Input: part model. Units: mm. Frame: model coordinates. A direction names the side the tool comes from. Round coordinates to 2 decimals unless told otherwise and drop trailing zeros. Loops run counter-clockwise (first coordinate to the right, second up) from the corner with the lowest first, then second, coordinate; pieces in that order, holes last. Notation, with made-up numbers: (38.5, 21) -> (61.5, 21) arc R25 ccw to (61.5, 37) -> close; hole circle Ø5 at (-34, -8.5). An arc over 180 degrees is marked (long way). Answer as a JSON object with one key per item and string values. Group by question number.
Item 1: Section query A-A on z = 0. Count the separate pieces of the cut face and the enclosed holes in it, and give its area (3 significant figures).
Item 2: Section query D-D on z = 2. Return loops of the section in (x, y).
Item 3: Section query C-C on x = 0.75. Return loops of the section in (y, z).
Item 4: Pin query (flat end, axial travel): pin 1 (1 mm diameter, centred on x = 3, z = -3, fed in from +Y); pin 2 (1.3 mm diameter, centred on x = -3.5, y = 5, fed in from +Z); pin 3 (2.5 mm diameter, centred on x = -2.5, z = 0, fed in from +Y). Return the tip coordinate at first contact, or that it passes through.
Item 5: Section query B-B on y = 3. Return loops of the section in (x, z), and give its area (3 significant figures).
Item 6: Draft query along Z for faces 4 (the flat face through (-5.004, 5, 0)), 5 (the flat face through (-2, 7.468, 0)), 6 (the cylindrical face through (3.144, -1.252, 0.084)). Return one class per face: released by +Z, released by -Z, zero draft, split by the parting line, or undercut.
Item 7: Material intervals for line 1 (X direction, y = 3.25, z = 0); line 2 (Y direction, x = 4.5, z = 1); line 3 (Y direction, x = -3.5, z = 0), sorted ascending. Write a range as [from, to].
Item 8: Set-up query: faces 1 (the flat face through (2, 6.604, 1)), 2 (the cylindrical face through (4.013, 8.755, -0.198)), 3 (the flat face through (-0.07, 8.45, 3.05)). Return all of +Z, -Z, +X, -X, +Y, -Y with unobstructed straight access to the full face (end or side cutting, diameter ignored); none if empty.
from build123d import *

# Parameters (mm, degrees)
SKETCH3_W                     = 10.0076
SKETCH3_H                     = 7.7978
BOSS_EXTRUDE1_DEPTH           = 10.0076
CUT_EXTRUDE1_DEPTH            = 10.0076
SKETCH5_R                     = 1.524
CUT_EXTRUDE2_DEPTH            = 2.54
SKETCH6_W                     = 4.4958
SKETCH6_H                     = 6.35
CUT_EXTRUDE3_DEPTH            = 5.08
SKETCH8_R                     = 0.6477
BOSS_EXTRUDE2_DEPTH           = 2.54
SKETCH9_R                     = 0.6477
BOSS_EXTRUDE3_DEPTH           = 0.9652
BOSS_EXTRUDE3_DRAFT           = 17
BOSS_EXTRUDE3_PROFILE_2_DEPTH = 0.9652
BOSS_EXTRUDE3_PROFILE_2_DRAFT = 17


with BuildPart() as part:
    # Sketch3 → Boss-Extrude1 (new body)
    with BuildSketch(Plane(origin=(0, 0, 0), x_dir=(1, 0, 0), z_dir=(0, 1, 0))):
        Rectangle(SKETCH3_W, SKETCH3_H)
    extrude(amount=BOSS_EXTRUDE1_DEPTH)

    # Sketch4 → Cut-Extrude1 (cut)
    with BuildSketch(Plane.ZY.offset(5.0038)):
        Polygon((-3.8989, 10.0076), (-3.8989, 6.858), (-2.2225, 10.0076), align=None)
        Polygon((3.8989, 10.0076), (2.2225, 10.0076), (3.8989, 6.858), align=None)
    extrude(amount=-CUT_EXTRUDE1_DEPTH, mode=Mode.SUBTRACT)

    # Sketch5 → Cut-Extrude2 (cut)
    with BuildSketch(Plane(origin=(0, 10.0076, 0), x_dir=(1, 0, 0), z_dir=(0, 1, 0))):
        with Locations(Location((-2.5019, 0, 0), (0, 0, 270))):
            Circle(SKETCH5_R)
        with Locations(Location((2.5019, 0, 0), (0, 0, 270))):
            Circle(SKETCH5_R)
    extrude(amount=-CUT_EXTRUDE2_DEPTH, mode=Mode.SUBTRACT)

    # Sketch6 → Cut-Extrude3 (cut)
    with BuildSketch(Plane.XY.offset(3.8989)):
        with Locations((-2.5019, 3.429)):
            Rectangle(SKETCH6_W, SKETCH6_H)
        with Locations((2.5019, 3.429)):
            Rectangle(SKETCH6_W, SKETCH6_H)
    extrude(amount=-CUT_EXTRUDE3_DEPTH, mode=Mode.SUBTRACT)

    # Sketch8 → Boss-Extrude2 (add)
    with BuildSketch(Plane.XZ):
        with Locations(Location((-2.5019, 0, 0), (0, 0, 270))):
            Circle(SKETCH8_R)
        with Locations(Location((2.5019, 0, 0), (0, 0, 270))):
            Circle(SKETCH8_R)
    extrude(amount=BOSS_EXTRUDE2_DEPTH)


with BuildPart() as boss_extrude3_tool:
    # Sketch9 → Boss-Extrude3 (with draft: the straight prism first)
    with BuildSketch(Plane.XZ.offset(2.54)):
        with Locations(Location((2.5019, 0, 0), (0, 0, 270))):
            Circle(SKETCH9_R)
    extrude(amount=BOSS_EXTRUDE3_DEPTH)
    # Boss-Extrude3: the draft: its side faces are tilted about the plane it starts from
    boss_extrude3_sides = [boss_extrude3_tool.faces().sort_by_distance(p)[0] for p in [
        (2.5019, -3.0226, 0.6477),
    ]]
    draft(boss_extrude3_sides, Plane.XZ.offset(2.54), BOSS_EXTRUDE3_DRAFT)


with BuildPart() as part_1:
    add(part.part)

    # Boss-Extrude3: add boss_extrude3_tool
    add(boss_extrude3_tool.part)


with BuildPart() as boss_extrude3_profile_2_tool:
    # Sketch9 → Boss-Extrude3 profile 2 (with draft: the straight prism first)
    with BuildSketch(Plane.XZ.offset(2.54)):
        with Locations(Location((-2.5019, 0, 0), (0, 0, 270))):
            Circle(SKETCH9_R)
    extrude(amount=BOSS_EXTRUDE3_PROFILE_2_DEPTH)
    # Boss-Extrude3 profile 2: the draft: its side faces are tilted about the plane it starts from
    boss_extrude3_profile_2_sides = [boss_extrude3_profile_2_tool.faces().sort_by_distance(p)[0] for p in [
        (-2.5019, -3.0226, 0.6477),
    ]]
    draft(boss_extrude3_profile_2_sides, Plane.XZ.offset(2.54), BOSS_EXTRUDE3_PROFILE_2_DRAFT)


with BuildPart() as part_2:
    add(part_1.part)

    # Boss-Extrude3 profile 2: add boss_extrude3_profile_2_tool
    add(boss_extrude3_profile_2_tool.part)


solid = part_2.part
Solved:
{
 "1": {"separate pieces": "1", "enclosed holes": "2", "area": "36.1 mm²"},
 "2": {"outline": "(-5, 0) -> (5, 0) -> (5, 10.01) -> (-5, 10.01) -> close; hole (-4.75, 0.25) -> (-0.25, 0.25) -> (-0.25, 6.6) -> (-4.75, 6.6) -> close; hole (0.25, 0.25) -> (4.75, 0.25) -> (4.75, 6.6) -> (0.25, 6.6) -> close"},
 "3": {"outline": "(0, -3.9) -> (6.86, -3.9) -> (10.01, -2.22) -> (10.01, 2.22) -> (6.86, 3.9) -> (6.6, 3.9) -> (6.6, -1.18) -> (0.25, -1.18) -> (0.25, 3.9) -> (0, 3.9) -> close"},
 "4": {"pin 1": "y = 9.49", "pin 2": "z = -1.18", "pin 3": "y = 7.47"},
 "5": {"outline": "(-5, -3.9) -> (5, -3.9) -> (5, 3.9) -> (4.75, 3.9) -> (4.75, -1.18) -> (0.25, -1.18) -> (0.25, 3.9) -> (-0.25, 3.9) -> (-0.25, -1.18) -> (-4.75, -1.18) -> (-4.75, 3.9) -> (-5, 3.9) -> close", "area": "32.4 mm²"},
 "6": {"face 4": "zero draft", "face 5": "undercut", "face 6": "split by the parting line"},
 "7": {"line 1": "[-5, -4.75], [-0.25, 0.25], [4.75, 5]", "line 2": "[0, 0.25], [6.6, 10.01]", "line 3": "[0, 0.25], [6.6, 7.47]"},
 "8": {"face 1": "+Z", "face 2": "+Y", "face 3": "+Z, +X, -X, +Y"}
}
